Verification items for this drawing (mm, ordinates from the low corner). Round coordinates to 2 decimals unless told otherwise and drop trailing zeros. Write each loop counter-clockwise with the first axis right and the second up, starting at its lowest first coordinate (ties: lowest second). Pieces come first, ordered by that corner, then holes. Notation, with made-up numbers: (44, 28.5) -> (86, 28.5) arc R23 cw to (86, 37.5) -> close; hole circle Ø1 at (57, 21). An arc over 180 degrees is marked (long way). Put each result on its own line as item: value. Start each with the question number.
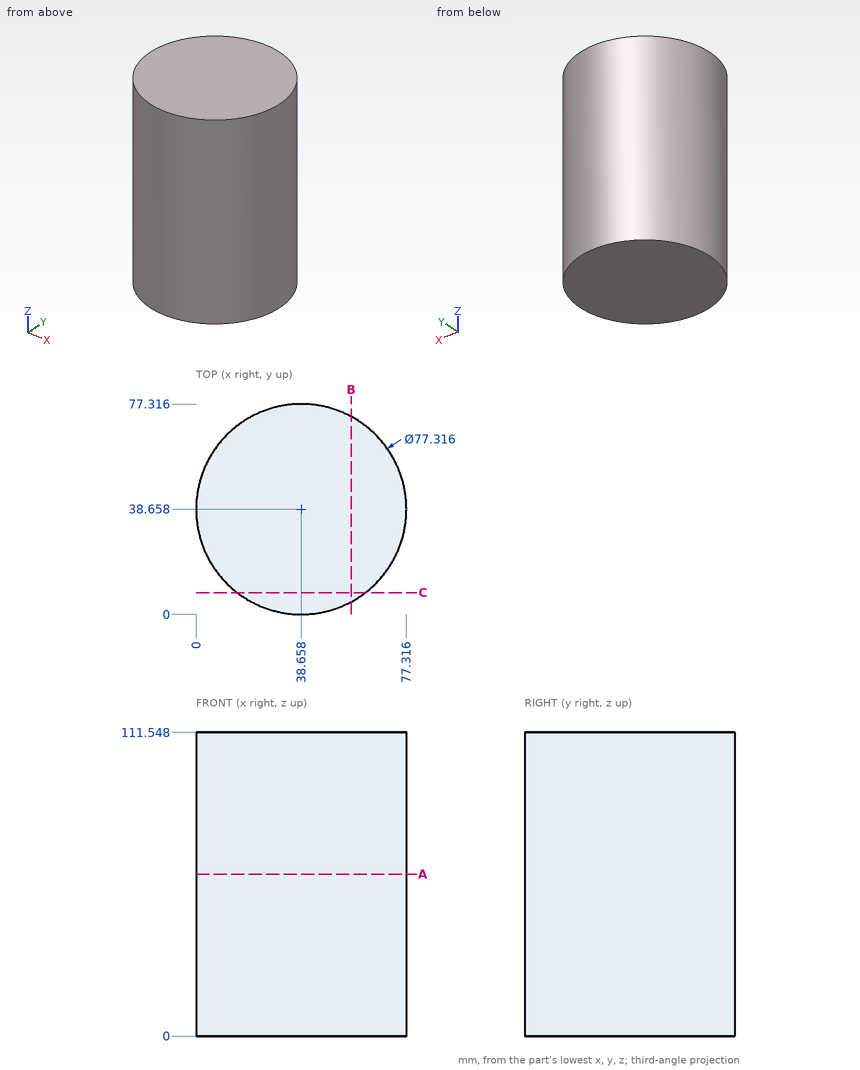
(1) Material ranges on L1, parallel to X at y = 40, z = 45; L2, parallel to X at y = 17, z = 29.5; L3, parallel to Y at x = 61, z = 51 (1 decimal), recorded low to high. Write a range as from..to.
(2) Sectioned sample at A-A (z = 59.5). Record the cut outline in (x, y), and give its area (4 significant figures).
(3) Go/stop test with flat-tipped pins: pin 1 Ø8 at (x, z) = (40.5, 62.5) entering from +Y; pin 2 Ø1.5 at (y, z) = (9.5, 52.5) entering from -X; pin 3 Ø1.5 at (y, z) = (31.5, 30.5) entering from +X. Record where each tip stops, or that it passes through.
(4) Sectioned sample at C-C (y = 8). Record the cut outline in (x, z), and give its area (3 significant figures).
(5) Sectioned sample at B-B (x = 57). Record the cut outline in (y, z).
Found:
1. L1: 0.02..77.29
1. L2: 6.64..70.68
1. L3: 7.1..70.2
2. outline: circle Ø77.32 at (38.66, 38.66)
2. area: 4,695 mm2
3. pin 1: y = 77.32
3. pin 2: x = 12.44
3. pin 3: x = 76.78
4. outline: (15.11, 0) -> (62.21, 0) -> (62.21, 111.55) -> (15.11, 111.55) -> close
4. area: 5,250 mm2
5. outline: (4.63, 0) -> (72.69, 0) -> (72.69, 111.55) -> (4.63, 111.55) -> close
